Autodesk Inventor part; units mm, degrees
ref_plane "YZ Plane" through (0, 0, 0) normal (1, 0, 0) x (0, 1, 0)
ref_plane "XZ Plane" through (0, 0, 0) normal (0, 1, 0) x (-1, 0, 0)
ref_plane "XY Plane" through (0, 0, 0) normal (0, 0, 1) x (1, 0, 0)
sketch "Sketch1" plane through (0, 0, 0) normal (0, 0, 1) x (1, 0, 0)
  line L0 (-25, -26) -> (25, -26)
  line L1 (25, -26) -> (25, 26)
  line L2 (25, 26) -> (-25, 26)
  line L3 (-25, 26) -> (-25, -26)
  line L4 (-25, -26) -> (25, 26) construction
  line L5 (25, -26) -> (-25, 26) construction
  circle A0 centre (0, 0) radius 4
  line L6 (-2.6458, -3) -> (2.6458, -3)
  line L7 (-45, 2.5) -> (-5, 2.5)
  line L8 (-5, 2.5) -> (-5, -2.5)
  line L9 (-5, -2.5) -> (-45, -2.5)
  line L10 (-45, -2.5) -> (-45, 2.5)
  line L11 (-45, 2.5) -> (-5, -2.5) construction
  line L12 (-5, 2.5) -> (-45, -2.5) construction
  point P0 (-25, 0)
  point P1 (-25, -2.5)
  point P2 (-25, 2.5)
  dimension "d0" = 50
  dimension "d1" = 52
  dimension "d2" = 8
  dimension "d39" = 3
  dimension "d40" = 20
  dimension "d41" = 5
extrude "Extrusion1" add sketch "Sketch1" along normal blind 10 contours L3 L9 L8 L7 L2 L1 L0 | L9 L10 L7 L3 | L3 L7 L8 L9 | L6 A0 picked at (-0.6179, -3.1815)
sketch "Sketch2" plane through (-25, -26, 0) normal (0, -1, 0) x (1, 0, 0)
  line L0 (0, 0) -> (0, 10)
  line L1 (50, 0) -> (50, 10)
  line L2 (0, 0) -> (50, 0)
  point P0 (25, 0)
  point P1 (0, 5)
  point P2 (45, 5)
  point P3 (25, 5)
  point P4 (5, 5)
  point P5 (0, 5)
  point P6 (50, 5)
  point P7 (25, 0)
  dimension "d19" = 5
  dimension "d20" = 5
hole "Hole1" at (20, -26, 5) at (-20, -26, 5) direction (0, 1, 0) diameter 3.242 depth 15 tip angle 118 countersink diameter 4 countersink angle 90
fillet "Fillet2" radius 0.5 8 edges at (0, 4, 10) (-25, -26, 5) (25, -26, 5) (25, 26, 5) (-25, 26, 5) (0, 4, 0) (0, -3, 10) (0, -3, 0)
hole "Hole2" at (0, -26, 5) direction (0, 1, 0) diameter 3.242 end up to surface countersink diameter 4 countersink angle 90
mirror "Mirror1" about plane through (0, 0, 0) normal (0, 1, 0) of "Hole1"
sketch "Sketch3" plane through (25, -25.5, 0.5) normal (1, 0, 0) x (0, 0, -1)
  line L0 (-9.5, 51) -> (0.5, 51)
  point P0 (0.5, 25.5)
  point P1 (-4.5, 25.5)
  point P2 (-4.5, 51)
  point P3 (-9, 51)
  point P4 (0, 51)
hole "Hole3" at (25, 0, 5) direction (-1, 0, 0) diameter 3.242 end up to surface countersink diameter 4 countersink angle 90
fillet "Fillet3" radius 2 2 edges at (-45, 2.5, 5) (-45, -2.5, 5)
fillet "Fillet4" radius 5 2 edges at (-25, -2.5, 5) (-25, 2.5, 5)
properties part number "bevestegingsKoppeling axis4_5" material "Aluminum 6061"
Geometry: final body of the model. Coordinates: model frame, mm. A direction names the side the tool comes from. Coordinates: 2 decimals unless noted, no trailing zeros. Order: outer loops, then holes, each group sorted by start corner. A loop starts at its lowest first (then second) coordinate and runs counter-clockwise, first axis right, second up.
(1) Section query C-C (x = 9.5). Return the cut outline in (y, z).
(2) Material intervals for probe 1 along X at (y, z) = (21.5, 5); probe 2 along Z at (x, y) = (0, -15.75); probe 3 along X at (y, z) = (-19.5, 5), sorted ascending.
(3) Draft query along X for faces 1 (the face through (-20.19, 10.195, 5.207)), 2 (the face through (-26.5, 3.93, 5.07)), 3 (the face through (-36, -2.5, 5)). Return one class per face: pulls with the +X half, pulls with the -X half, needs draft (parallel to the pull), parting line crosses it, or undercut.
(4) Section query B-B (x = 0). Return the cut outline in (y, z).
(5) Section query D-D (x = -40). Return the cut outline in (y, z), plus the area to 3 significant figures.
(6) Access query for faces 4 (the face through (-18.418, -18.208, 5.351)), 5 (the face through (-37, 2.5, 5)), 6 (the face through (13.99, -0.07, 6.62)), 7 (the face through (18.418, 18.208, 5.351)). Directions: +Z, -Z, +X, -X, +Y, -Y. A direction counts if a zero-diameter tool reaches every point of the face in a straight line with its end or side. Return the directions, or none.
(7) Section query A-A (y = -22). Return the cut outline in (x, z), plus the area to 3 significant figures.
(8) First-contact query: pin 1 (2.5 mm diameter, centred on x = 20, z = 5, fed in from -Y); pin 2 (3 mm diameter, centred on x = -20, z = 5, fed in from -Y); pin 3 (3 mm diameter, centred on y = 0, z = 5, fed in from +X); pin 4 (2 mm diameter, centred on x = 11.5, y = -17.5, fed in from -Z). Flat tips, straight axial feed; report the tip coordinate or a pass-through.
Solution:
1. outline: (-26, 0) - (26, 0) - (26, 10) - (-26, 10) - close; hole circle Ø3.24 at (0, 5)
2. probe 1: x = -25 to -21.62, -18.38 to 18.38, 21.62 to 25
2. probe 2: z = 0 to 3.38, 6.62 to 10
2. probe 3: x = -25 to -21.62, -18.38 to -1.62, 1.62 to 18.38, 21.62 to 25
3. face 1: undercut
3. face 2: pulls with the -X half
3. face 3: needs draft
4. outline: (-26, 0) - (-3.5, 0) arc R0.5 ccw to (-3, 0.5) - (-3, 3.38) - (-25.62, 3.38) - (-26, 3) - close; (-26, 7) - (-25.62, 6.62) - (-3, 6.62) - (-3, 9.5) arc R0.5 ccw to (-3.5, 10) - (-26, 10) - close; (4, 0.5) arc R0.5 ccw to (4.5, 0) - (26, 0) - (26, 10) - (4.5, 10) arc R0.5 ccw to (4, 9.5) - close
5. outline: (-2.5, 0) - (2.5, 0) - (2.5, 10) - (-2.5, 10) - close
5. area: 50.0 mm2
6. face 4: -Y
6. face 5: +Z, -Z, -X, +Y
6. face 6: +X
6. face 7: +Y
7. outline: (-25, 0) - (25, 0) - (25, 10) - (-25, 10) - close; hole circle Ø3.24 at (-20, 5); hole circle Ø3.24 at (0, 5); hole circle Ø3.24 at (20, 5)
7. area: 475 mm2
8. pin 1: stops at y = -10.78
8. pin 2: stops at y = -10.93
8. pin 3: stops at x = -3.71
8. pin 4: stops at z = 0
